Input: dimensioned drawing with shaded views. Units: mm. Origin: part minimum x, y, z. A direction names the side the tool comes from. Give positions to 0.01 mm unless a question says otherwise; leave off trailing zeros. Loops run counter-clockwise (first coordinate to the right, second up) from the corner with the lowest first, then second, coordinate; pieces in that order, holes last. Notation, with made-up numbers: (5, 59.25) -> (22, 59.25) arc R15 cw to (22, 88.25) -> close; hole circle Ø4 at (36.25, -11.5). An arc over 180 degrees is marked (long way). Answer as a JSON object with one key per item and string values.
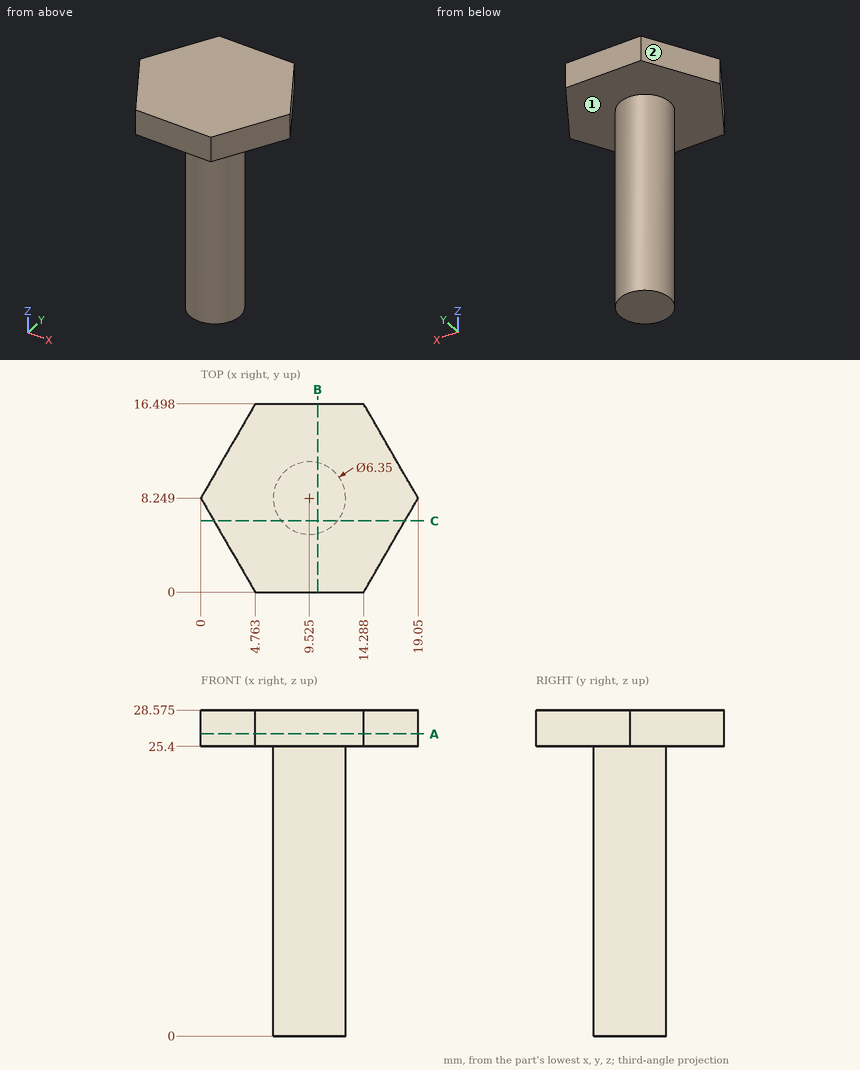
Q1. Section A-A, the plane z = 26.5. Return the cut outline in (x, y).
Evaluation:
{"outline": "(0, 8.25) -> (4.76, 0) -> (14.29, 0) -> (19.05, 8.25) -> (14.29, 16.5) -> (4.76, 16.5) -> close"}
Q2. Section B-B, the plane x = 10.25. Return the cut outline in (y, z) (1 decimal), then the cut area to 3 significant figures.
Evaluation:
{"outline": "(0, 25.4) -> (5.2, 25.4) -> (5.2, 0) -> (11.3, 0) -> (11.3, 25.4) -> (16.5, 25.4) -> (16.5, 28.6) -> (0, 28.6) -> close", "area": "209 mm2"}
Q3. Access query for the marked faces 1 and 2. Directions: +Z, -Z, +X, -X, +Y, -Y. A direction counts if a zero-diameter tool reaches every point of the face in a straight line with its end or side. Return the directions, or none.
Evaluation:
{"face 1": "-Z", "face 2": "+Z, -Z, -X, +Y"}
Q4. Ray query, line 1 along Z through (x, y) = (8.5, 3.25) (1 decimal); line 2 along X through (y, z) = (9, 22.5); line 3 along X through (y, z) = (6.75, 18) (1 decimal). Return the intervals inside material, ascending.
Evaluation:
{"line 1": "z = 25.4 to 28.6", "line 2": "x = 6.44 to 12.61", "line 3": "x = 6.7 to 12.3"}
Q5. Section C-C, the plane y = 6.25. Return the cut outline in (x, z) (1 decimal).
Evaluation:
{"outline": "(1.2, 25.4) -> (7.1, 25.4) -> (7.1, 0) -> (12, 0) -> (12, 25.4) -> (17.9, 25.4) -> (17.9, 28.6) -> (1.2, 28.6) -> close"}
Q6. Pin query (flat end, axial travel): pin 1 (6 mm diameter, centred on x = 2.5, z = 17.5, fed in from +Y); pin 2 (3 mm diameter, centred on x = 11, z = 15.5, fed in from -Y); pin 3 (8 mm diameter, centred on y = 7, z = 10.5, fed in from -X). Return the tip coordinate at first contact, or that it passes through.
Evaluation:
{"pin 1": "passes through", "pin 2": "stops at y = 5.07", "pin 3": "stops at x = 6.35"}
